from build123d import *

# Parameters (mm, degrees)
SKETCH1_W                = 115
SKETCH1_H                = 36.5
BOSS_EXTRUDE1_DEPTH      = 1
BOSS_EXTRUDE2_DEPTH      = 20
BOSS_EXTRUDE2_DEPTH_BACK = 1
SKETCH2_W                = 119
SKETCH2_H                = 40.5
SKETCH2_W_2              = 115
SKETCH2_H_2              = 36.5
SKETCH3_R                = 1.5
SKETCH3_W                = 6
SKETCH3_H                = 6
BOSS_EXTRUDE3_DEPTH      = 4
SKETCH4_R                = 1.5
SKETCH4_W                = 5.5
SKETCH4_H                = 6.495155074
BOSS_EXTRUDE4_DEPTH      = 13
SKETCH5_W                = 15
SKETCH5_H                = 10
CUT_EXTRUDE1_DEPTH       = 8
SKETCH6_W                = 46
SKETCH6_H                = 7.792677535
CUT_EXTRUDE2_DEPTH       = 8
SKETCH7_W                = 10.3
SKETCH7_H                = 10.3
CUT_EXTRUDE3_DEPTH       = 8
SKETCH8_W                = 15
SKETCH8_H                = 5
CUT_EXTRUDE4_DEPTH       = 8
SKETCH9_W                = 119
SKETCH9_H                = 40.5
SKETCH9_W_2              = 17
SKETCH9_H_2              = 17
SKETCH9_W_3              = 73
SKETCH9_H_3              = 26
BOSS_EXTRUDE5_DEPTH      = 3
CUT_EXTRUDE5_DEPTH       = 10
CUT_EXTRUDE5_DEPTH_BACK  = 10
SKETCH10_R               = 1.5


with BuildPart() as part:
    # Sketch1 → Boss-Extrude1 (new body)
    with BuildSketch(Plane(origin=(0, 0, 0), x_dir=(1, 0, 0), z_dir=(0, 1, 0))):
        Rectangle(SKETCH1_W, SKETCH1_H)
    extrude(amount=BOSS_EXTRUDE1_DEPTH)


with BuildPart() as body_2:
    # Sketch2 → Boss-Extrude2 (new, two sides: drawn at the far end of the back side and taken through both)
    with BuildSketch(Plane(origin=(0, 1, 0), x_dir=(1, 0, 0), z_dir=(0, 1, 0)).offset(-BOSS_EXTRUDE2_DEPTH_BACK)):
        Rectangle(SKETCH2_W, SKETCH2_H)
        Rectangle(SKETCH2_W_2, SKETCH2_H_2, mode=Mode.SUBTRACT)
    extrude(amount=BOSS_EXTRUDE2_DEPTH + BOSS_EXTRUDE2_DEPTH_BACK)

    # Intersect1: read off the stored shape, not the designer's step
    # Intersect1: union part
    add(part.part)

    # Sketch3 → Boss-Extrude3 (add)
    # profile 1 of 4: a face of its own
    with BuildSketch(Plane(origin=(0, 1, 0), x_dir=(1, 0, 0), z_dir=(0, 1, 0))):
        Polygon((-51.5, 7.25), (-51.5, 13.25), (-54, 13.25), (-57.5, 13.25), (-57.5, 9.75), (-57.5, 7.25), align=None)
        with Locations(Location((-54, 9.75, 0), (0, 0, 270))):
            Circle(SKETCH3_R, mode=Mode.SUBTRACT)
    # profile 2 of 4: a face of its own
    with BuildSketch(Plane(origin=(0, 1, 0), x_dir=(1, 0, 0), z_dir=(0, 1, 0))):
        with Locations((-25.5, 10.25)):
            Rectangle(SKETCH3_W, SKETCH3_H)
        with Locations(Location((-26, 9.75, 0), (0, 0, 90))):
            Circle(SKETCH3_R, mode=Mode.SUBTRACT)
    # profile 3 of 4: a face of its own
    with BuildSketch(Plane(origin=(0, 1, 0), x_dir=(1, 0, 0), z_dir=(0, 1, 0))):
        with Locations((-25.5, -10.25)):
            Rectangle(SKETCH3_W, SKETCH3_H)
        with Locations(Location((-26, -9.75, 0), (0, 0, 270))):
            Circle(SKETCH3_R, mode=Mode.SUBTRACT)
    # profile 4 of 4: a face of its own
    with BuildSketch(Plane(origin=(0, 1, 0), x_dir=(1, 0, 0), z_dir=(0, 1, 0))):
        with Locations((-54.5, -10.25)):
            Rectangle(SKETCH3_W, SKETCH3_H)
        with Locations(Location((-54, -9.75, 0), (0, 0, 90))):
            Circle(SKETCH3_R, mode=Mode.SUBTRACT)
    extrude(amount=BOSS_EXTRUDE3_DEPTH)

    # Sketch4 → Boss-Extrude4 (add)
    # profile 1 of 4: a face of its own
    with BuildSketch(Plane(origin=(0, 1, 0), x_dir=(1, 0, 0), z_dir=(0, 1, 0))):
        Polygon((-22.5, 13.25), (-22.5, 11.754844926), (-17, 11.754844926), (-17, 18.25), (-20, 18.25), (-22.5, 18.25), (-22.5, 15.25), align=None)
        with Locations(Location((-20, 15.25, 0), (0, 0, 90))):
            Circle(SKETCH4_R, mode=Mode.SUBTRACT)
    # profile 2 of 4: a face of its own
    with BuildSketch(Plane(origin=(0, 1, 0), x_dir=(1, 0, 0), z_dir=(0, 1, 0))):
        with Locations((-19.75, -15.002422463)):
            Rectangle(SKETCH4_W, SKETCH4_H)
        with Locations(Location((-20, -15.25, 0), (0, 0, 90))):
            Circle(SKETCH4_R, mode=Mode.SUBTRACT)
    # profile 3 of 4: a face of its own
    with BuildSketch(Plane(origin=(0, 1, 0), x_dir=(1, 0, 0), z_dir=(0, 1, 0))):
        with Locations((54.75, -15.002422463)):
            Rectangle(SKETCH4_W, SKETCH4_H)
        with Locations(Location((55, -15.25, 0), (0, 0, 90))):
            Circle(SKETCH4_R, mode=Mode.SUBTRACT)
    # profile 4 of 4: a face of its own
    with BuildSketch(Plane(origin=(0, 1, 0), x_dir=(1, 0, 0), z_dir=(0, 1, 0))):
        with Locations((54.75, 15.002422463)):
            Rectangle(SKETCH4_W, SKETCH4_H)
        with Locations(Location((55, 15.25, 0), (0, 0, 90))):
            Circle(SKETCH4_R, mode=Mode.SUBTRACT)
    extrude(amount=BOSS_EXTRUDE4_DEPTH)

    # Sketch5 → Cut-Extrude1 (cut)
    with BuildSketch(Plane.ZY.offset(59.5)):
        with Locations((0, 11.525411997)):
            Rectangle(SKETCH5_W, SKETCH5_H)
    extrude(amount=-CUT_EXTRUDE1_DEPTH, mode=Mode.SUBTRACT)

    # Sketch6 → Cut-Extrude2 (cut)
    with BuildSketch(Plane(origin=(0, 0, -20.25), x_dir=(-1, 0, 0), z_dir=(0, 0, -1))):
        with Locations((-6.5, 11.396338768)):
            Rectangle(SKETCH6_W, SKETCH6_H)
    extrude(amount=-CUT_EXTRUDE2_DEPTH, mode=Mode.SUBTRACT)

    # Sketch7 → Cut-Extrude3 (cut)
    with BuildSketch(Plane.XY.offset(20.25)):
        with Locations((-49.05, 10.55)):
            Rectangle(SKETCH7_W, SKETCH7_H)
    extrude(amount=-CUT_EXTRUDE3_DEPTH, mode=Mode.SUBTRACT)

    # Sketch8 → Cut-Extrude4 (cut)
    with BuildSketch(Plane(origin=(0, 0, -20.25), x_dir=(-1, 0, 0), z_dir=(0, 0, -1))):
        with Locations((40.794043984, 3.5)):
            Rectangle(SKETCH8_W, SKETCH8_H)
    extrude(amount=-CUT_EXTRUDE4_DEPTH, mode=Mode.SUBTRACT)

    # Sketch10 → Cut-Extrude5 (cut, two sides: drawn at the far end of the back side and taken through both)
    with BuildSketch(Plane(origin=(0, 1, 0), x_dir=(1, 0, 0), z_dir=(0, 1, 0)).offset(-CUT_EXTRUDE5_DEPTH_BACK)):
        with Locations(Location((55, 15.25, 0), (0, 0, 90))):
            Circle(SKETCH10_R)
        with Locations(Location((55, -15.25, 0), (0, 0, 90))):
            Circle(SKETCH10_R)
        with Locations(Location((-54, -9.75, 0), (0, 0, 90))):
            Circle(SKETCH10_R)
        with Locations(Location((-20, -15.25, 0), (0, 0, 90))):
            Circle(SKETCH10_R)
        with Locations(Location((-26, -9.75, 0), (0, 0, 90))):
            Circle(SKETCH10_R)
        with Locations(Location((-20, 15.25, 0), (0, 0, 90))):
            Circle(SKETCH10_R)
        with Locations(Location((-26, 9.75, 0), (0, 0, 90))):
            Circle(SKETCH10_R)
        with Locations(Location((-54, 9.75, 0), (0, 0, 90))):
            Circle(SKETCH10_R)
    extrude(amount=CUT_EXTRUDE5_DEPTH + CUT_EXTRUDE5_DEPTH_BACK, mode=Mode.SUBTRACT)


with BuildPart() as body_2_2:
    # Sketch9 → Boss-Extrude5 (new body)
    with BuildSketch(Plane(origin=(0, 21, 0), x_dir=(1, 0, 0), z_dir=(0, 1, 0))):
        Rectangle(SKETCH9_W, SKETCH9_H)
        with Locations((-40, 1.75)):
            Rectangle(SKETCH9_W_2, SKETCH9_H_2, mode=Mode.SUBTRACT)
        with Locations((17.25, -0.25)):
            Rectangle(SKETCH9_W_3, SKETCH9_H_3, mode=Mode.SUBTRACT)
    extrude(amount=BOSS_EXTRUDE5_DEPTH)


solid = body_2.part
The model under review builds one solid part; all positions refer to its coordinate system, in mm. A direction names the side the tool comes from. Round coordinates to 2 decimals unless told otherwise and drop trailing zeros. Write each loop counter-clockwise with the first axis right and the second up, starting at its lowest first coordinate (ties: lowest second). Pieces come first, ordered by that corner, then holes. Notation, with made-up numbers: M 2,8 L 7,8 A16 ccw 7,17 Z; hole C 57.5,29.25 d3. An arc over 180 degrees is marked long. Use a Markdown table: item, result. Add a question column.
Q1. The part is to be moulded in two halves that separate along Y. For faces 1 (the face through (-24, 5, 10)), 2 (the face through (7, 15.293, -19)), 3 (the face through (59.5, 10, 0)), say which applies: pulls with the +Y half, pulls with the -Y half, needs draft (parallel to the pull), parting line crosses it, or undercut.
Q2. We need section D-D, the plane z = 3.5. State the section outline as (x, y) points.
Q3. To check wall thickness, follow line 1 (X direction, y = 12.05, z = 15.25); line 2 (Z direction, x = 55, y = 11); line 3 (Z direction, x = -30, y = 8). State the ranges of each line that lie inside material, in increasing order.
Q4. Insertion check: pin 1 (6 mm diameter, centred on x = -19, z = 13.5, fed in from +Y); pin 2 (5 mm diameter, centred on x = -17, z = -14.5, fed in from -Y); pin 3 (1.8 mm diameter, centred on x = -54, z = 9.75, fed in from -Y); pin 4 (8 mm diameter, centred on x = 12, z = -9, fed in from +Y). Each pin has a flat end and moves straight along its axis. Give the tip position at first contact, or say it passes through.
Q5. We need section A-A, the plane x = 2.5. State the section outline as (y, z) points, plus the area to 3 significant figures.
Q6. Machinability: for faces 4 (the face through (-18, 21, -20)), 5 (the face through (-49, 5.4, 19)), 6 (the face through (-1, 11, 18.25)), 7 (the face through (-33.294, 3, -19)), which of the approach directions +Z, -Z, +X, -X, +Y, -Y give a long, thin tool a straight path to every point of the face, cutting with its end or side? Answer none if there is none.
Q7. We need section C-C, the plane x = 55. State the section outline as (y, z) points.
Q8. We need section B-B, the plane z = -15.25. State the section outline as (x, y) points, plus the area to 3 significant figures.
Findings below:
| question | item | result |
|---|---|---|
| 1 | face 1 | pulls with the +Y half |
| 1 | face 2 | undercut |
| 1 | face 3 | needs draft |
| 2 | outline | M -59.5,0 L 59.5,0 L 59.5,21 L 57.5,21 L 57.5,1 L -57.5,1 L -57.5,6.53 L -59.5,6.53 Z; M -59.5,16.53 L -57.5,16.53 L -57.5,21 L -59.5,21 Z |
| 3 | line 1 | x = -59.5 to -57.5, -22.5 to -21.5, -18.5 to -17, 52 to 53.5, 56.5 to 59.5 |
| 3 | line 2 | z = -20.25 to -16.75, -13.75 to -11.75, 11.75 to 13.75, 16.75 to 20.25 |
| 3 | line 3 | z = -20.25 to -18.25, 18.25 to 20.25 |
| 4 | pin 1 | stops at y = 14 |
| 4 | pin 2 | stops at y = 0 |
| 4 | pin 3 | passes through |
| 4 | pin 4 | stops at y = 1 |
| 5 | outline | M 0,-20.25 L 7.5,-20.25 L 7.5,-18.25 L 1,-18.25 L 1,18.25 L 21,18.25 L 21,20.25 L 0,20.25 Z; M 15.29,-20.25 L 21,-20.25 L 21,-18.25 L 15.29,-18.25 Z |
| 5 | area | 105 mm² |
| 6 | face 4 | +Z, -Z, +X, -X, +Y |
| 6 | face 5 | +Z |
| 6 | face 6 | +Y |
| 6 | face 7 | -Z |
| 7 | outline | M 0,-20.25 L 21,-20.25 L 21,-18.25 L 14,-18.25 L 14,-16.75 L 0,-16.75 Z; M 0,-13.75 L 14,-13.75 L 14,-11.75 L 1,-11.75 L 1,11.75 L 14,11.75 L 14,13.75 L 0,13.75 Z; M 0,16.75 L 14,16.75 L 14,18.25 L 21,18.25 L 21,20.25 L 0,20.25 Z |
| 8 | outline | M -59.5,0 L -21.5,0 L -21.5,14 L -22.5,14 L -22.5,1 L -57.5,1 L -57.5,21 L -59.5,21 Z; M -18.5,0 L 53.5,0 L 53.5,14 L 52,14 L 52,1 L -17,1 L -17,14 L -18.5,14 Z; M 56.5,0 L 59.5,0 L 59.5,21 L 57.5,21 L 57.5,14 L 56.5,14 Z |
| 8 | area | 258 mm² |
